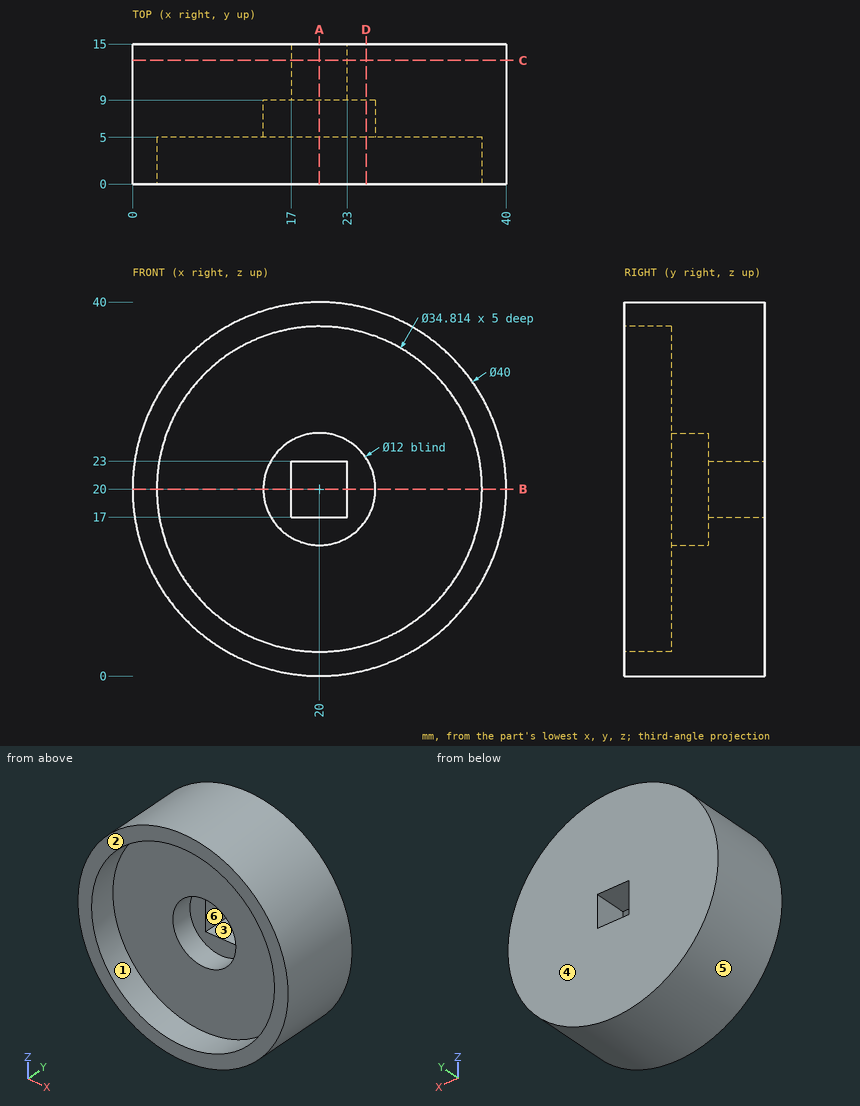
The figure shows three views and two pictorial views of one solid part (mm, origin at its lowest corner). Answer the questions. A direction names the side the tool comes from. Round coordinates to 2 decimals unless told otherwise and drop trailing zeros. Write each loop counter-clockwise with the first axis right and the second up, starting at its lowest first coordinate (ties: lowest second). Pieces come first, ordered by that corner, then holes. Notation, with made-up numbers: (-1, 50) - (49, 50) arc R8 ccw to (49, 65) - close; hole circle Ø1 at (-24, 4.5). An arc over 180 degrees is marked (long way). Answer in a Markdown table with one row per item. Add a question column.
1. A cutting plane is placed at A-A, the plane x = 20. Determine the outline of the cut face in (y, z), and give its area (3 significant figures).
2. A cutting plane is placed at C-C, the plane y = 13.25. Determine the outline of the cut face in (x, z).
3. Given pin 1 (5 mm diameter, centred on x = 34, z = 23.5, fed in from -Y); pin 2 (6 mm diameter, centred on x = 9.5, y = 12, fed in from -Z); pin 3 (5 mm diameter, centred on x = 16, y = 9, fed in from +Z); pin 4 (5 mm diameter, centred on y = 13, z = 20.5, fed in from -X), each flat-ended and moving along its own axis, determine where each tip first touches the part or whether it passes through.
4. The mould has two halves that part along X. Classify the marked faces 4, 5 and 6: +X half, -X half, draft (parallel to the pull), parting line (faces both ways), or undercut.
5. A cutting plane is placed at B-B, the plane z = 20. Determine the outline of the cut face in (x, y).
6. A cutting plane is placed at D-D, the plane x = 25. Determine the outline of the cut face in (y, z) (1 decimal).
7. Find the intervals of material crossed by line 1 along Z through (x, y) = (20, 1.4); line 2 along X through (y, z) = (11.25, 20.5); line 3 along Y through (x, z) = (33, 16), in increasing order. Write a range as from..to.
8. For the marked faces 1, 2 and 3, determine the directions among +Z, -Z, +X, -X, +Y, -Y from which every point of the face is accessible in a straight line to the end or side of a thin tool.
Worked out:
| question | item | result |
|---|---|---|
| 1 | outline | (0, 0) - (15, 0) - (15, 17) - (9, 17) - (9, 14) - (5, 14) - (5, 2.59) - (0, 2.59) - close; (0, 37.41) - (5, 37.41) - (5, 26) - (9, 26) - (9, 23) - (15, 23) - (15, 40) - (0, 40) - close |
| 1 | area | 342 mm^2 |
| 2 | outline | circle Ø40 at (20, 20); hole (17, 17) - (23, 17) - (23, 23) - (17, 23) - close |
| 3 | pin 1 | y = 5 |
| 3 | pin 2 | z = 1.46 |
| 3 | pin 3 | z = 39.94 |
| 3 | pin 4 | x = 0 |
| 4 | face 4 | draft |
| 4 | face 5 | parting line |
| 4 | face 6 | undercut |
| 5 | outline | (0, 0) - (2.59, 0) - (2.59, 5) - (14, 5) - (14, 9) - (17, 9) - (17, 15) - (0, 15) - close; (23, 9) - (26, 9) - (26, 5) - (37.41, 5) - (37.41, 0) - (40, 0) - (40, 15) - (23, 15) - close |
| 6 | outline | (0, 0.6) - (15, 0.6) - (15, 39.4) - (0, 39.4) - (0, 36.7) - (5, 36.7) - (5, 23.3) - (9, 23.3) - (9, 16.7) - (5, 16.7) - (5, 3.3) - (0, 3.3) - close |
| 7 | line 1 | 0..2.59, 37.41..40 |
| 7 | line 2 | 0.01..17, 23..39.99 |
| 7 | line 3 | 5..15 |
| 8 | face 1 | -Y |
| 8 | face 2 | +Z, -Z, +X, -X, -Y |
| 8 | face 3 | +Y, -Y |
